from build123d import *

# Parameters (mm, degrees)
SKETCH1_W            = 25.7
SKETCH1_H            = 16
BOSS_EXTRUDE5_DEPTH  = 13
SKETCH3_W            = 24
SKETCH3_H            = 10
CUT_EXTRUDE1_DEPTH   = 12
SKETCH6_W            = 6
SKETCH6_H            = 12
CUT_EXTRUDE6_DEPTH   = 12
SKETCH12_W           = 25.7
SKETCH12_H           = 13
CUT_EXTRUDE9_DEPTH   = 1
SKETCH13_W           = 25.7
SKETCH13_H           = 13
CUT_EXTRUDE10_DEPTH  = 1
SKETCH14_W           = 25.7
SKETCH14_H           = 0.24
CUT_EXTRUDE11_DEPTH  = 26.979383268
SKETCH15_W           = 25.7
SKETCH15_H           = 0.24
BOSS_EXTRUDE6_DEPTH  = 13
BOSS_EXTRUDE8_DEPTH  = 10
SKETCH19_R           = 2.35
CUT_EXTRUDE12_DEPTH  = 29.801827185
SKETCH20_R           = 2.4
SKETCH20_R_2         = 2.45
BOSS_EXTRUDE9_DEPTH  = 2.5
SKETCH21_R           = 1.5
CUT_EXTRUDE13_DEPTH  = 29.801827185
SKETCH22_W           = 10
SKETCH22_H           = 14
BOSS_EXTRUDE11_DEPTH = 13
SKETCH25_W           = 8
SKETCH25_H           = 10
CUT_EXTRUDE17_DEPTH  = 12
SKETCH26_W           = 1.5
SKETCH26_H           = 2
BOSS_EXTRUDE12_DEPTH = 13
SKETCH27_W           = 0.5
SKETCH27_H           = 1.76
SKETCH27_W_2         = 0.500587584
SKETCH27_H_2         = 2
CUT_EXTRUDE18_DEPTH  = 12
SKETCH28_W           = 1.277363426
SKETCH28_H           = 0.860849325
BOSS_EXTRUDE13_DEPTH = 12
CUT_EXTRUDE20_DEPTH  = 12


with BuildPart() as part:
    # Sketch1 → Boss-Extrude5 (new body)
    with BuildSketch(Plane(origin=(0, 0, 0), x_dir=(1, 0, 0), z_dir=(0, 1, 0))):
        with Locations((4.864219333, 6.861269364)):
            Rectangle(SKETCH1_W, SKETCH1_H)
    extrude(amount=BOSS_EXTRUDE5_DEPTH)

    # Sketch3 → Cut-Extrude1 (cut)
    with BuildSketch(Plane(origin=(0, 13, 0), x_dir=(1, 0, 0), z_dir=(0, 1, 0))):
        with Locations((5.015394501, 6.623768503)):
            Rectangle(SKETCH3_W, SKETCH3_H)
    extrude(amount=-CUT_EXTRUDE1_DEPTH, mode=Mode.SUBTRACT)

    # Sketch6 → Cut-Extrude6 (cut)
    with BuildSketch(Plane.ZY.offset(7.985780667)):
        with Locations((-6.861269364, 7)):
            Rectangle(SKETCH6_W, SKETCH6_H)
    extrude(amount=-CUT_EXTRUDE6_DEPTH, mode=Mode.SUBTRACT)

    # Sketch12 → Cut-Extrude9 (cut)
    with BuildSketch(Plane(origin=(0, 0, -14.861269364), x_dir=(-1, 0, 0), z_dir=(0, 0, -1))):
        with Locations((-4.864219333, 6.5)):
            Rectangle(SKETCH12_W, SKETCH12_H)
    extrude(amount=-CUT_EXTRUDE9_DEPTH, mode=Mode.SUBTRACT)

    # Sketch13 → Cut-Extrude10 (cut)
    with BuildSketch(Plane.XY.offset(1.138730636)):
        with Locations((4.864219333, 6.5)):
            Rectangle(SKETCH13_W, SKETCH13_H)
    extrude(amount=-CUT_EXTRUDE10_DEPTH, mode=Mode.SUBTRACT)

    # Sketch14 → Cut-Extrude11 (cut, through all)
    with BuildSketch(Plane(origin=(0, 13, 0), x_dir=(1, 0, 0), z_dir=(0, 1, 0))):
        with Locations((4.864219333, 13.741269364)):
            Rectangle(SKETCH14_W, SKETCH14_H)
    extrude(amount=-CUT_EXTRUDE11_DEPTH, mode=Mode.SUBTRACT)

    # Sketch15 → Boss-Extrude6 (add)
    with BuildSketch(Plane(origin=(0, 13, 0), x_dir=(1, 0, 0), z_dir=(0, 1, 0))):
        with Locations((4.864219333, -0.258730636)):
            Rectangle(SKETCH15_W, SKETCH15_H)
    extrude(amount=-BOSS_EXTRUDE6_DEPTH)

    # Sketch17 → Boss-Extrude8 (add)
    with BuildSketch(Plane(origin=(17.714219333, 0, 0), x_dir=(0, 0, -1), z_dir=(1, 0, 0))):
        with BuildLine():
            Line((13.621269364, 13), (18.621269364, 13))
            Line((18.621269364, 13), (18.621269364, 9))
            add(Edge.make_bspline(
                [(18.621269364, 9), (13.621269364, 9), (13.621269364, 6.5)],
                knots=[0, 0, 0, 1, 1, 1], degree=2))
            Line((13.621269364, 6.5), (13.621269364, 13))
        make_face()
        with BuildLine():
            Line((-0.378730636, 13), (-5.378730636, 13))
            Line((-5.378730636, 13), (-5.378730636, 9))
            add(Edge.make_bspline(
                [(-5.378730636, 9), (-0.378730636, 9), (-0.378730636, 6.5)],
                knots=[0, 0, 0, 1, 1, 1], degree=2))
            Line((-0.378730636, 6.5), (-0.378730636, 13))
        make_face()
    extrude(amount=-BOSS_EXTRUDE8_DEPTH)

    # Sketch19 → Cut-Extrude12 (cut, through all)
    with BuildSketch(Plane(origin=(0, 13, 0), x_dir=(1, 0, 0), z_dir=(0, 1, 0))):
        with Locations(Location((12.714219333, 15.871269364, 0), (0, 0, 270))):
            Circle(SKETCH19_R)
        with Locations(Location((12.714219333, -2.628730636, 0), (0, 0, 270))):
            Circle(SKETCH19_R)
    extrude(amount=-CUT_EXTRUDE12_DEPTH, mode=Mode.SUBTRACT)

    # Sketch20 → Boss-Extrude9 (add)
    with BuildSketch(Plane(origin=(0, 13, 0), x_dir=(1, 0, 0), z_dir=(0, 1, 0))):
        with Locations((12.714219333, 15.871269364)):
            Circle(SKETCH20_R)
        with Locations((12.714219333, -2.628730636)):
            Circle(SKETCH20_R_2)
    extrude(amount=-BOSS_EXTRUDE9_DEPTH)

    # Sketch21 → Cut-Extrude13 (cut, through all)
    with BuildSketch(Plane(origin=(0, 13, 0), x_dir=(1, 0, 0), z_dir=(0, 1, 0))):
        with Locations(Location((12.714219333, 15.871269364, 0), (0, 0, 270))):
            Circle(SKETCH21_R)
        with Locations(Location((12.714219333, -2.628730636, 0), (0, 0, 270))):
            Circle(SKETCH21_R)
    extrude(amount=-CUT_EXTRUDE13_DEPTH, mode=Mode.SUBTRACT)

    # Sketch22 → Boss-Extrude11 (add)
    with BuildSketch(Plane(origin=(0, 13, 0), x_dir=(1, 0, 0), z_dir=(0, 1, 0))):
        with Locations((-12.985780667, 6.621269364)):
            Rectangle(SKETCH22_W, SKETCH22_H)
    extrude(amount=-BOSS_EXTRUDE11_DEPTH)

    # Sketch25 → Cut-Extrude17 (cut)
    with BuildSketch(Plane(origin=(0, 13, 0), x_dir=(1, 0, 0), z_dir=(0, 1, 0))):
        with Locations((-11.985780667, 6.621269364)):
            Rectangle(SKETCH25_W, SKETCH25_H)
    extrude(amount=-CUT_EXTRUDE17_DEPTH, mode=Mode.SUBTRACT)

    # Sketch26 → Boss-Extrude12 (add)
    with BuildSketch(Plane(origin=(0, 13, 0), x_dir=(1, 0, 0), z_dir=(0, 1, 0))):
        with Locations((-8.234605499, 2.623768503)):
            Rectangle(SKETCH26_W, SKETCH26_H)
        with Locations((-8.234605499, 10.623768503)):
            Rectangle(SKETCH26_W, SKETCH26_H)
    extrude(amount=-BOSS_EXTRUDE12_DEPTH)

    # Sketch27 → Cut-Extrude18 (cut)
    with BuildSketch(Plane(origin=(0, 13, 0), x_dir=(1, 0, 0), z_dir=(0, 1, 0))):
        with Locations((-7.234605499, 10.741269364)):
            Rectangle(SKETCH27_W, SKETCH27_H)
        Polygon((-7.985780667, 3.861269364), (-7.985780667, 3.623768503), (-7.485193083, 3.623768503), (-6.984605499, 3.623768503), (-6.984605499, 3.861269364), align=None)
        with Locations((-7.234899291, 2.623768503)):
            Rectangle(SKETCH27_W_2, SKETCH27_H_2)
    extrude(amount=-CUT_EXTRUDE18_DEPTH, mode=Mode.SUBTRACT)

    # Sketch28 → Boss-Extrude13 (add)
    with BuildSketch(Plane(origin=(0, 13, 0), x_dir=(1, 0, 0), z_dir=(0, 1, 0))):
        with Locations((-8.345923786, 1.388186548)):
            Rectangle(SKETCH28_W, SKETCH28_H)
    extrude(amount=-BOSS_EXTRUDE13_DEPTH)

    # Sketch35 → Cut-Extrude20 (cut)
    with BuildSketch(Plane(origin=(17.714219333, 0, 0), x_dir=(0, 0, -1), z_dir=(1, 0, 0))):
        with BuildLine():
            Line((4.421384975, 7), (4.421384975, 13))
            Line((4.421384975, 13), (8.821153753, 13))
            Line((8.821153753, 13), (8.821153753, 7))
            ThreePointArc((8.821153753, 7), (6.621269364, 4.800115611), (4.421384975, 7))
        make_face()
    extrude(amount=-CUT_EXTRUDE20_DEPTH, mode=Mode.SUBTRACT)


solid = part.part
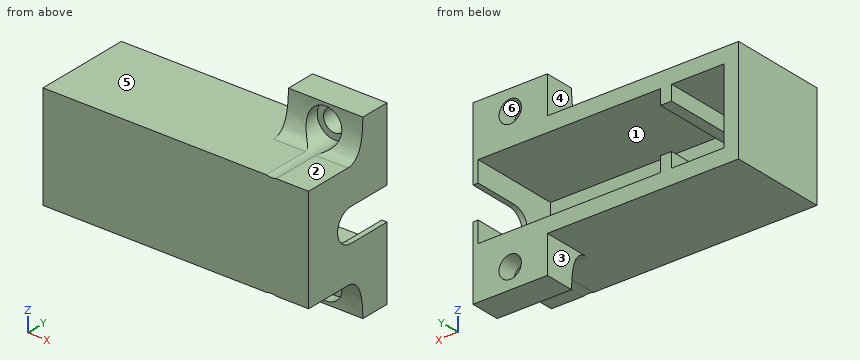
Work out the finished part from the listing and answer in its coordinate system (mm). Face numbers are marked on the shaded views. A direction names the side the tool comes from. Coordinates: 2 decimals unless noted, no trailing zeros. Loops run counter-clockwise (first coordinate to the right, second up) from the corner with the lowest first, then second, coordinate; pieces in that order, holes last. Notation, with made-up numbers: (72, 41.5) -> (121, 41.5) arc R25 cw to (121, 62.5) -> close; hole circle Ø11 at (27, 7.5). An arc over 180 degrees is marked (long way). Write each question's results on one line, items separated by ' | '. Start each with the question number.
1) Consider line 1 along X through (y, z) = (9, -10.25); line 2 along Z through (x, y) = (-14, 10.25); line 3 along X through (y, z) = (10.75, -4.25). Determine where each line is inside the solid, lowest interval first.
2) For the marked faces 1, 2 and 3, determine the directions among +Z, -Z, +X, -X, +Y, -Y from which every point of the face is accessible in a straight line to the end or side of a thin tool.
3) The mould has two halves that part along Z. Classify the marked faces 4, 5 and 6: pulls with the +Z half, pulls with the -Z half, needs draft (parallel to the pull), parting line crosses it, or undercut.
4) Find section B-B on z = -2. Determine the outline of the cut face in (x, y), then the cut area to 3 significant figures.
5) Find section C-C on y = 11.75. Count the separate pieces of the cut face and the enclosed holes in it, then the cut area to 3 significant figures.
6) Flat-ended cylindrical pins translate along their axes: P1, Ø1, axis at x = -13.5, z = -11.5, coming from the -Y side; P2, Ø1, axis at x = 10.5, z = 1.5, coming from the -Y side; P3, Ø4, axis at x = 4.5, y = 5, coming from the -Z side; P4, Ø4, axis at x = 12.71, z = 2.63, coming from the -Y side. Find the tip coordinate at first contact, or state that the pin passes through.
7) Find section D-D on x = -6. Determine the outline of the cut face in (y, z).
Response values:
1) line 1: x = -17.99 to -15.99, -8.98 to -7.48, 17.02 to 17.71 | line 2: z = -13.62 to -11.62, -1.62 to 0.38 | line 3: x = -17.99 to -15.99, 17.02 to 17.71
2) face 1: +Y | face 2: +Z, +X, -X, -Y | face 3: -Z, -X, +Y, -Y
3) face 4: needs draft | face 5: pulls with the +Z half | face 6: undercut
4) outline: (-17.99, 0) -> (17.71, 0) -> (17.71, 13) -> (17.02, 13) -> (17.02, 1) -> (-7.49, 1) -> (-7.49, 13) -> (-8.98, 13) -> (-8.98, 1) -> (-15.99, 1) -> (-15.99, 13) -> (-17.99, 13) -> close | area: 86.1 mm^2
5) separate pieces: 1 | enclosed holes: 2 | area: 259 mm^2
6) P1: stops at y = 0 | P2: stops at y = 7.95 | P3: stops at z = -13.62 | P4: stops at y = 10.5
7) outline: (0, -13.62) -> (13, -13.62) -> (13, -11.62) -> (1, -11.62) -> (1, -1.62) -> (13, -1.62) -> (13, 0.38) -> (0, 0.38) -> close
